CAD build for the part. Positions are in the model's coordinates, mm. A direction names the side the tool comes from. Give positions to 0.01 mm unless a question says otherwise; leave off trailing zeros. Loops run counter-clockwise (first coordinate to the right, second up) from the corner with the lowest first, then second, coordinate; pieces in that order, holes last. Notation, with made-up numbers: (4.25, 9.25) - (17.25, 9.25) arc R18 cw to (17.25, 13.25) - close; hole circle Ø9 at (79.5, -9). An arc over 180 degrees is marked (long way). Return JSON: item names as keys, results as strings.
from build123d import *

# Parameters (mm, degrees)
BOSS_EXTRUDE1_DEPTH            = 18.75
CBORE_FOR_M5_SHCS2_D           = 5.5
CBORE_FOR_M5_SHCS2_CBORE_D     = 10
CBORE_FOR_M5_SHCS2_CBORE_DEPTH = 6
CUT_EXTRUDE1_DEPTH             = 350
CUT_EXTRUDE2_DEPTH             = 12.1
SKETCH30_R                     = 2.5
CUT_EXTRUDE3_DEPTH             = 252.935329003


with BuildPart() as part:
    # Sketch1 → Boss-Extrude1 (new body)
    with BuildSketch(Plane.XY):
        Polygon((90, 22), (90, -210), (90, -235), (-90, -235), (-90, 165), (90, 165), align=None)
    extrude(amount=BOSS_EXTRUDE1_DEPTH)

    # CBORE for M5 SHCS2 (through all)
    with Locations(Plane.XY.offset(18.75)):
        with Locations((-60.75, -200), (-60.75, -168), (-24.75, -168), (-24.75, -200), (24.75, -200), (24.75, -168), (60.75, -168), (60.75, -200), (-60.75, -20), (-60.75, 12), (-24.75, -20), (24.75, 12), (60.75, 12), (60.75, -20), (24.75, -20), (-24.75, 12)):
            CounterBoreHole(CBORE_FOR_M5_SHCS2_D / 2, CBORE_FOR_M5_SHCS2_CBORE_D / 2, CBORE_FOR_M5_SHCS2_CBORE_DEPTH)

    # Sketch28 → Cut-Extrude1 (cut)
    with BuildSketch(Plane(origin=(0, 165, 0), x_dir=(1, 0, 0), z_dir=(0, 1, 0))):
        Polygon((23.074976608, -18.75), (17.946938328, -13.621961721), (13.555789015, -10.796343736), (-13.555789015, -10.796343736), (-17.946938328, -13.621961721), (-23.074976608, -18.75), align=None)
    extrude(amount=-CUT_EXTRUDE1_DEPTH, mode=Mode.SUBTRACT)

    # Sketch29 → Cut-Extrude2 (cut)
    with BuildSketch(Plane.XY.offset(18.75)):
        Polygon((0, 165), (37.5, 165), (37.5, 133), (-37.5, 133), (-37.5, 165), align=None)
    extrude(amount=-CUT_EXTRUDE2_DEPTH, mode=Mode.SUBTRACT)

    # Sketch30 → Cut-Extrude3 (cut, through all)
    with BuildSketch(Plane.XY.offset(6.65)):
        with Locations((23, 159)):
            Circle(SKETCH30_R)
        with Locations((-23, 159)):
            Circle(SKETCH30_R)
        with Locations((23, 146)):
            Circle(SKETCH30_R)
        with Locations((-23, 146)):
            Circle(SKETCH30_R)
    extrude(amount=-CUT_EXTRUDE3_DEPTH, mode=Mode.SUBTRACT)


solid = part.part
1. Cut at B-B, the plane x = -7. Write the cut outline in (y, z).
Values follow:
{"outline": "(-235, 0) - (165, 0) - (165, 6.65) - (133, 6.65) - (133, 10.8) - (-185, 10.8) - (-185, 18.75) - (-235, 18.75) - close"}
2. Cut at A-A, the plane y = -86. Write the cut outline in (x, z), plus the area to 3 significant figures.
Values follow:
{"outline": "(-90, 0) - (90, 0) - (90, 18.75) - (23.07, 18.75) - (17.95, 13.62) - (13.56, 10.8) - (-13.56, 10.8) - (-17.95, 13.62) - (-23.07, 18.75) - (-90, 18.75) - close", "area": "3,080 mm²"}
3. Drop flat-ended pins along their axis: P1, Ø1.5, axis at x = -21, y = -6, coming from the +Z side (3 decimals); P2, Ø6, axis at x = -23, y = 146, coming from the +Z side; P3, Ø9, axis at x = 60.75, y = -200, coming from the +Z side. Give the stop position or say it passes through.
Values follow:
{"P1": "stops at z = 17.425", "P2": "stops at z = 6.65", "P3": "stops at z = 12.75"}
4. Pull direction Y, two halves, no side cores. Call faces 3 (the face through (-29.745, 12.22, 15.792)), 4 (the face through (-90, -38, 9)), 5 (the face through (1, 133, 10)): +Y half, -Y half, draft (parallel to the pull), parting line (faces both ways), or undercut.
Values follow:
{"face 3": "undercut", "face 4": "draft", "face 5": "+Y half"}
5. Drill centre lines: probe 1 along Y at (x, z) = (-24.75, 15.3); probe 2 along Y at (x, z) = (60.75, 3.5); probe 3 along X at (y, z) = (-141, 16.25). Where is each one in solid material? Low to high.
Values follow:
{"probe 1": "y = -235 to -205, -195 to -173, -163 to -25, -15 to 7, 17 to 133", "probe 2": "y = -235 to -202.75, -197.25 to -170.75, -165.25 to -22.75, -17.25 to 9.25, 14.75 to 165", "probe 3": "x = -90 to -20.57, 20.57 to 90"}
6. Which spindle directions (+Z, -Z, +X, -X, +Y, -Y) get a long thin tool onto all of the face, cutting with end or side? Do faces 1 (the face through (1, -32, 0)), 2 (the face through (-58.6, 9.8, 12.75)). Say none if no direction does.
Values follow:
{"face 1": "-Z, +X, -X, +Y, -Y", "face 2": "+Z"}
